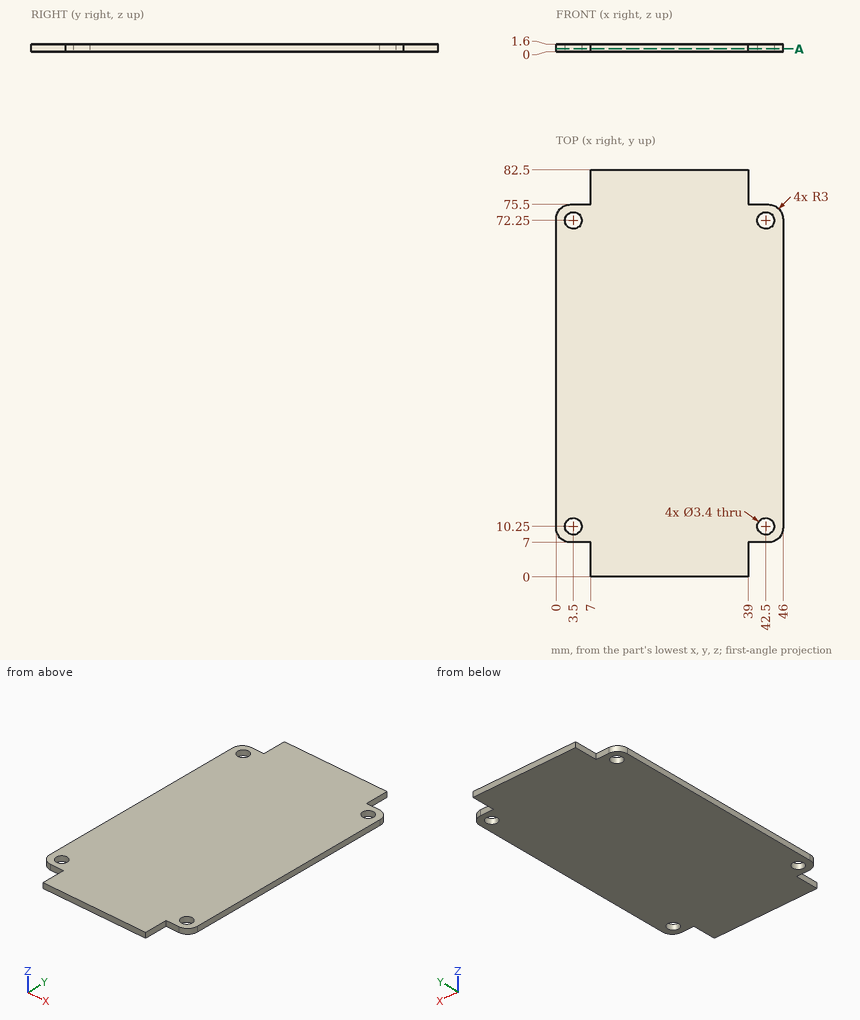
Drawing for the job (mm, zero at the part's lowest x, y, z). Round coordinates to 2 decimals unless told otherwise and drop trailing zeros. Write each loop counter-clockwise with the first axis right and the second up, starting at its lowest first coordinate (ties: lowest second). Pieces come first, ordered by that corner, then holes.
Item 1: Drill centre lines: L1, parallel to Y at x = 42.5, z = 1.15; L2, parallel to X at y = 72.25, z = 0.4; L3, parallel to X at y = 71, z = 0.35. Where is each one in solid material? Low to high.
Filled in:
L1: y = 7 to 8.55, 11.95 to 70.55, 73.95 to 75.5
L2: x = 0 to 1.8, 5.2 to 40.8, 44.2 to 46
L3: x = 0 to 2.35, 4.65 to 41.35, 43.65 to 46
Item 2: Band-saw the part on A-A on z = 0.6. Write the cut outline in (x, y), then the cut area to 3 significant figures.
Filled in:
outline: (0, 10) arc R3 ccw to (3, 7) - (7, 7) - (7, 0) - (39, 0) - (39, 7) - (43, 7) arc R3 ccw to (46, 10) - (46, 72.5) arc R3 ccw to (43, 75.5) - (39, 75.5) - (39, 82.5) - (7, 82.5) - (7, 75.5) - (3, 75.5) arc R3 ccw to (0, 72.5) - close; hole circle Ø3.4 at (3.5, 10.25); hole circle Ø3.4 at (3.5, 72.25); hole circle Ø3.4 at (42.5, 10.25); hole circle Ø3.4 at (42.5, 72.25)
area: 3,550 mm2
Item 3: Drop flat-ended pins along their axis: pin 1 Ø0.8 at (y, z) = (78.5, 1) entering from -X; pin 2 Ø0.8 at (y, z) = (2.5, 0.5) entering from +X; pin 3 Ø3 at (x, y) = (42.5, 72.25) entering from -Z; pin 4 Ø0.5 at (x, z) = (40, 1) entering from +Y. Give the stop position or say it passes through.
Filled in:
pin 1: stops at x = 7
pin 2: stops at x = 39
pin 3: passes through
pin 4: stops at y = 75.5
